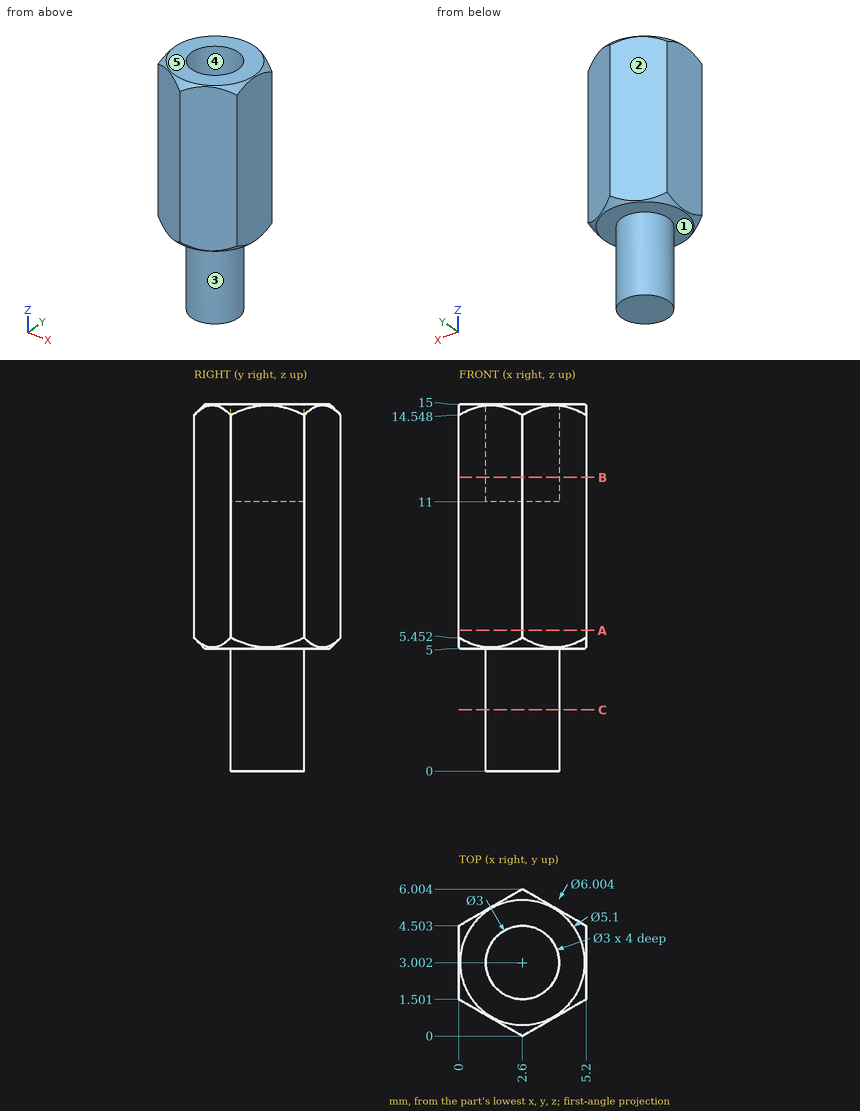
For this review, use the dimensioned drawing (mm, ordinates from the lowest corner) and the shaded views. A direction names the side the tool comes from. Round coordinates to 2 decimals unless told otherwise and drop trailing zeros. Order: outer loops, then holes, each group sorted by start corner. A loop starts at its lowest first (then second) coordinate and runs counter-clockwise, first axis right, second up. Notation, with made-up numbers: M -29.5,31 L 25.5,31 A20 cw 25.5,43 Z; hole C 33,29 d1. An arc over 180 degrees is marked long. Use a Markdown table: item, result.
1) Insertion check: pin 1 (2 mm diameter, centred on y = 4, z = 2, fed in from +X); pin 2 (1.5 mm diameter, centred on x = 3, y = 3.5, fed in from +Z); pin 3 (1.5 mm diameter, centred on x = 1, z = 3.5, fed in from -Y) (1 decimal). Each pin has a flat end and moves straight along its axis. Give the tip position at first contact, or say it passes through.
Report:
| item | result |
|---|---|
| pin 1 | x = 4.1 |
| pin 2 | z = 11 |
| pin 3 | y = 1.8 |
2) Wall thickness on line 1 along Z through (x, y) = (0.65, 3.25); line 2 along Z through (x, y) = (2.2, 4); line 3 along Y through (x, z) = (2.05, 7) (1 decimal): over which ranges is each line inside the solid? List them lowest first. Write a range as [from, to].
Report:
| item | result |
|---|---|
| line 1 | [5, 15] |
| line 2 | [0, 11] |
| line 3 | [0.3, 5.7] |
3) Tool access review of the marked faces 1 and 2: name each direction out of +Z, -Z, +X, -X, +Y, -Y from which nothing blocks a thin tool from reaching the whole face with its end or side.
Report:
| item | result |
|---|---|
| face 1 | -Z |
| face 2 | +Z, -Z, -X, +Y |
4) Consider section B-B (z = 12). Write out the cut boundary in (x, y) (1 decimal).
Report:
| item | result |
|---|---|
| outline | M 0,1.5 L 2.6,0 L 5.2,1.5 L 5.2,4.5 L 2.6,6 L 0,4.5 Z; hole C 2.6,3 d3 |
5) Consider section C-C (z = 2.5). Write out the cut boundary in (x, y).
Report:
| item | result |
|---|---|
| outline | C 2.6,3 d3 |
6) Draft analysis for pull direction Y (two halves, no side actions). For the marked faces 3, 4 and 5, state which applies: released by +Y, released by -Y, zero draft, split by the parting line, or undercut.
Report:
| item | result |
|---|---|
| face 3 | split by the parting line |
| face 4 | undercut |
| face 5 | zero draft |
7) Consider section A-A (z = 5.75). Write out the cut boundary in (x, y) (1 decimal).
Report:
| item | result |
|---|---|
| outline | M 0,1.5 L 2.6,0 L 5.2,1.5 L 5.2,4.5 L 2.6,6 L 0,4.5 Z |
